```python
from build123d import *

# Parameters (mm, degrees)
SKETCH_1_W      = 70
SKETCH_1_H      = 60
EXTRUDE_1_DEPTH = 55
SHELL_1_T       = -3
SKETCH_2_W      = 102
SKETCH_2_H      = 76
EXTRUDE_2_DEPTH = 3
FILLET_1_R      = 3
FILLET_4_R      = 3
EXTRUDE_3_DEPTH = 6
EXTRUDE_4_DEPTH = 3


with BuildPart() as part:
    # 草图1 → 凸台-拉伸1 (new body)
    with BuildSketch(Plane.XY):
        Rectangle(SKETCH_1_W, SKETCH_1_H)
    extrude(amount=EXTRUDE_1_DEPTH)

    # 抽壳1
    shell_1_openings = [part.faces().sort_by_distance(p)[0] for p in [
        (0, 30, 27.5),
    ]]
    offset(amount=SHELL_1_T, openings=shell_1_openings, kind=Kind.INTERSECTION)

    # 草图2 → 凸台-拉伸2 (add)
    with BuildSketch(Plane.XY.offset(55)):
        with Locations((0, 8)):
            Rectangle(SKETCH_2_W, SKETCH_2_H)
    extrude(amount=EXTRUDE_2_DEPTH)

    # 圆角1
    fillet_1_edges = [part.edges().sort_by_distance(p)[0] for p in [
        (0, 46, 58),
        (51, 8, 58),
        (0, -30, 58),
        (-51, 8, 58),
    ]]
    fillet(fillet_1_edges, radius=FILLET_1_R - 0.0001)  # a hair under: the kernel refuses the full size

    # 圆角4
    fillet_4_edges = [part.edges().sort_by_distance(p)[0] for p in [
        (0, -30, 0),
        (-35, 0, 0),
        (0, 30, 0),
        (35, 0, 0),
        (35, -30, 27.5),
        (-35, -30, 27.5),
        (-35, 30, 27.5),
        (35, 30, 27.5),
    ]]
    fillet(fillet_4_edges, radius=FILLET_4_R - 0.0001)  # a hair under: the kernel refuses the full size

    # 草图3 → 凸台-拉伸3 (add)
    with BuildSketch(Plane.XY.offset(58)):
        with BuildLine():
            Line((-10, 15.5), (10, 15.5))
            ThreePointArc((10, 15.5), (17.5, 8), (10, 0.5))
            Line((10, 0.5), (-10, 0.5))
            ThreePointArc((-10, 0.5), (-17.5, 8), (-10, 15.5))
        make_face()
    extrude(amount=EXTRUDE_3_DEPTH)

    # 草图4 → 凸台-拉伸4 (add)
    with BuildSketch(Plane.XY.offset(64)):
        with BuildLine():
            Line((-15, 17.5), (15, 17.5))
            ThreePointArc((15, 17.5), (24.5, 8), (15, -1.5))
            Line((15, -1.5), (-15, -1.5))
            ThreePointArc((-15, -1.5), (-24.5, 8), (-15, 17.5))
        make_face()
    extrude(amount=EXTRUDE_4_DEPTH)


solid = part.part
```
The listing builds one solid part. Answer for the finished solid, in the listing's coordinates (mm). A direction names the side the tool comes from. Give positions to 0.01 mm unless a question says otherwise; leave off trailing zeros.
1) Given P1, Ø14.5, axis at y = 9.5, z = 23.5, coming from the -X side; P2, Ø12, axis at x = 3.5, z = 12, coming from the +Y side; P3, Ø15.5, axis at y = -12.5, z = 18.5, coming from the +X side, each flat-ended and moving along its own axis, determine where each tip first touches the part or whether it passes through.
Reported:
P1: stops at x = -35
P2: stops at y = -27
P3: stops at x = 35
2) Consider line 1 along X through (y, z) = (-3, 6.5); line 2 along Z through (x, y) = (17, -20.5); line 3 along Z through (x, y) = (-7, 42). Determine where each line is inside the solid, lowest interval first.
Reported:
line 1: x = -35 to -32, 32 to 35
line 2: z = 0 to 3, 52 to 58
line 3: z = 55 to 58
3) Determine the mould class of faces 5 (the face through (0, 8, 67)), 6 (the face through (-34.1, -29.14, 29.36)), 7 (the face through (-17.5, 7.84, 60.96)) for opening direction Z: pulls with the +Z half, pulls with the -Z half, needs draft (parallel to the pull), parting line crosses it, or undercut.
Reported:
face 5: pulls with the +Z half
face 6: needs draft
face 7: undercut
4) For faces 1 (the face through (0, 15.5, 61)), 2 (the face through (17.5, 8.16, 60.96)), 3 (the face through (34.1, -29.14, 29.36)), 4 (the face through (-24.498, 7.791, 65.479)), determine the directions among +Z, -Z, +X, -X, +Y, -Y from which every point of the face is accessible in a straight line to the end or side of a thin tool.
Reported:
face 1: +X, -X, +Y
face 2: +X
face 3: -Z, +X, -Y
face 4: +Z, -X
